Work out the finished part from the listing and answer in its coordinate system (mm). Round coordinates to 2 decimals unless told otherwise and drop trailing zeros. Loops run counter-clockwise (first coordinate to the right, second up) from the corner with the lowest first, then second, coordinate; pieces in that order, holes last. Notation, with made-up numbers: (29, 24.25) - (70, 24.25) arc R37 ccw to (70, 62.25) - close; hole circle Ø5 at (34, 16.25). An arc over 180 degrees is marked (long way). Return JSON: item names as keys, results as strings.
from build123d import *

# Parameters (mm, degrees)
EXTRUDE_1_DEPTH = 4
FILLET_1_R      = 0.75


with BuildPart() as part:
    # Эскиз1 → Бобышка-Вытянуть1 (new body)
    with BuildSketch(Plane.XY):
        Polygon((-6.08, -3.25), (6.08, -3.25), (7.821669751, 3.25), (-7.821669751, 3.25), align=None)
    extrude(amount=EXTRUDE_1_DEPTH)

    # Скругление1
    fillet_1_edges = [part.edges().sort_by_distance(p)[0] for p in [
        (0, 3.25, 0),
        (6.950834875, 0, 0),
        (0, -3.25, 0),
        (-6.950834875, 0, 0),
        (-7.821669751, 3.25, 2),
        (7.821669751, 3.25, 2),
        (6.08, -3.25, 2),
        (-6.08, -3.25, 2),
    ]]
    fillet(fillet_1_edges, radius=FILLET_1_R)


solid = part.part
1) Flat-ended cylindrical pins translate along their axes: pin 1 (1 mm diameter, centred on y = 1.5, z = 1.5, fed in from +X); pin 2 (1.5 mm diameter, centred on y = -1.5, z = 1.5, fed in from +X). Find the tip coordinate at first contact, or state that the pin passes through.
Verdict:
{"pin 1": "stops at x = 7.49", "pin 2": "stops at x = 6.75"}
2) Find the intervals of material crossed by L1, parallel to X at y = 0, z = 0.3; L2, parallel to X at y = -2.5, z = 3.75; L3, parallel to Y at x = 4, z = 0.65, in increasing order.
Verdict:
{"L1": "x = -6.8 to 6.8", "L2": "x = -6.28 to 6.28", "L3": "y = -3.24 to 3.24"}
3) Section A-A (z = 1.55) is taken. Give the vertices of the cut face in (x, y).
Verdict:
{"outline": "(-7.57, 2.31) - (-6.23, -2.69) arc R0.75 ccw to (-5.5, -3.25) - (5.5, -3.25) arc R0.75 ccw to (6.23, -2.69) - (7.57, 2.31) arc R0.75 ccw to (6.84, 3.25) - (-6.84, 3.25) arc R0.75 ccw to start"}
